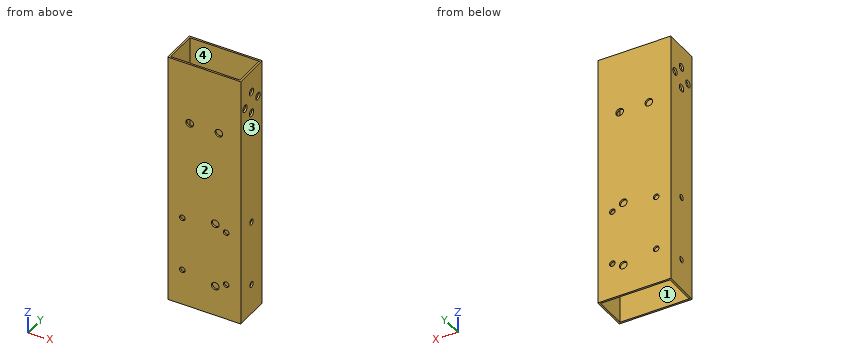
from build123d import *

# Parameters (mm, degrees)
SKETCH_1_W          = 40
SKETCH_1_H          = 20
SKETCH_1_W_2        = 38
SKETCH_1_H_2        = 18
EXTRUDE_1_DEPTH     = 140
SKETCH_2_R          = 2
SKETCH_2_R_2        = 1.55
CUT_EXTRUDE_1_DEPTH = 147.969384567
SKETCH_3_R          = 1.55
SKETCH_3_R_2        = 2.1
CUT_EXTRUDE_2_DEPTH = 147.969384567
SKETCH_4_R          = 2.1
CUT_EXTRUDE_3_DEPTH = 147.969384567


with BuildPart() as part:
    # 草图1 → 凸台-拉伸1 (new body)
    with BuildSketch(Plane.XY):
        with Locations((20, 10)):
            Rectangle(SKETCH_1_W, SKETCH_1_H)
        with Locations((20, 10)):
            Rectangle(SKETCH_1_W_2, SKETCH_1_H_2, mode=Mode.SUBTRACT)
    extrude(amount=EXTRUDE_1_DEPTH)

    # 草图2 → 切除-拉伸1 (cut, through all)
    with BuildSketch(Plane(origin=(0, 0, 0), x_dir=(0, 0, -1), z_dir=(1, 0, 0))):
        with Locations(Location((-116, 10, 0), (0, 0, 180))):
            Circle(SKETCH_2_R)
        with Locations(Location((-128, 10, 0), (0, 0, 180))):
            Circle(SKETCH_2_R)
        with Locations(Location((-16.8, 10, 0), (0, 0, 180))):
            Circle(SKETCH_2_R_2)
        with Locations(Location((-52.8, 10, 0), (0, 0, 180))):
            Circle(SKETCH_2_R_2)
        with Locations(Location((-122, 16, 0), (0, 0, 180))):
            Circle(SKETCH_2_R)
        with Locations(Location((-122, 4, 0), (0, 0, 180))):
            Circle(SKETCH_2_R)
    extrude(amount=CUT_EXTRUDE_1_DEPTH, mode=Mode.SUBTRACT)

    # 草图3 → 切除-拉伸2 (cut, through all)
    with BuildSketch(Plane(origin=(0, 0, 0), x_dir=(1, 0, 0), z_dir=(0, 1, 0))):
        with Locations(Location((8, -19.9, 0), (0, 0, 90))):
            Circle(SKETCH_3_R)
        with Locations(Location((32, -19.9, 0), (0, 0, 90))):
            Circle(SKETCH_3_R)
        with Locations(Location((32, -49.9, 0), (0, 0, 90))):
            Circle(SKETCH_3_R)
        with Locations(Location((8, -49.9, 0), (0, 0, 90))):
            Circle(SKETCH_3_R)
        with Locations(Location((26, -16.9, 0), (0, 0, 90))):
            Circle(SKETCH_3_R_2)
        with Locations(Location((26, -52.9, 0), (0, 0, 90))):
            Circle(SKETCH_3_R_2)
    extrude(amount=CUT_EXTRUDE_2_DEPTH, mode=Mode.SUBTRACT)

    # 草图4 → 切除-拉伸3 (cut, through all)
    with BuildSketch(Plane(origin=(0, 20, 0), x_dir=(1, 0, 0), z_dir=(0, 1, 0))):
        with Locations(Location((28, -106, 0), (0, 0, 270))):
            Circle(SKETCH_4_R)
        with Locations(Location((12, -106, 0), (0, 0, 270))):
            Circle(SKETCH_4_R)
    extrude(amount=-CUT_EXTRUDE_3_DEPTH, mode=Mode.SUBTRACT)


solid = part.part
The model under review builds one solid part; all positions refer to its coordinate system, in mm. Face numbers are marked on the shaded views. Give positions to 0.01 mm unless a question says otherwise; leave off trailing zeros. Write each loop counter-clockwise with the first axis right and the second up, starting at its lowest first coordinate (ties: lowest second). Pieces come first, ordered by that corner, then holes. Notation, with made-up numbers: M 55,-21.75 L 98,-21.75 A12 ccw 98,-6.75 Z; hole C -26,9 d6. An arc over 180 degrees is marked long. One line per question, with ' | ' between items. Start each with the question number.
Item 1: We need section D-D on z = 102.5. Write out the cut boundary in (x, y), plus the area to 3 significant figures.
Item 2: We need section B-B on z = 122. Write out the cut boundary in (x, y).
Item 3: For pin 1 (2 mm diameter, centred on y = 6, z = 15, fed in from -X), flat-tipped, find the tip position at first contact; note if it passes through.
Item 4: Draft analysis for pull direction X (two halves, no side actions). For the marked faces 1, 2, 3 and 4, state which applies: released by +X, released by -X, zero draft, split by the parting line, or undercut.
Item 5: We need section C-C on x = 8. Write out the cut boundary in (y, z), plus the area to 3 significant figures.
Item 6: Wall thickness on line 1 (X direction, y = 0.4, z = 106); line 2 (X direction, y = 6.5, z = 46); line 3 (X direction, y = 19.25, z = 49.9): over which ranges is each line inside the solid? List them lowest first. Write a range as from..to.
Item 7: We need section A-A on x = 36.5. Write out the cut boundary in (y, z).
Results found:
1) outline: M 0,0 L 40,0 L 40,20 L 0,20 Z; hole M 1,1 L 39,1 L 39,19 L 1,19 Z | area: 116 mm2
2) outline: M 0,0 L 40,0 L 40,2 L 39,2 L 39,1 L 1,1 L 1,2 L 0,2 Z; M 0,6 L 1,6 L 1,14 L 0,14 Z; M 0,18 L 1,18 L 1,19 L 39,19 L 39,18 L 40,18 L 40,20 L 0,20 Z; M 39,6 L 40,6 L 40,14 L 39,14 Z
3) pin 1: stops at x = 0
4) face 1: undercut | face 2: zero draft | face 3: released by +X | face 4: undercut
5) outline: M 0,0 L 1,0 L 1,18.35 L 0,18.35 Z; M 0,21.45 L 1,21.45 L 1,48.35 L 0,48.35 Z; M 0,51.45 L 1,51.45 L 1,140 L 0,140 Z; M 19,0 L 20,0 L 20,18.35 L 19,18.35 Z; M 19,21.45 L 20,21.45 L 20,48.35 L 19,48.35 Z; M 19,51.45 L 20,51.45 L 20,140 L 19,140 Z | area: 268 mm2
6) line 1: x = 0..9.9, 14.1..25.9, 30.1..40 | line 2: x = 0..1, 39..40 | line 3: x = 0..6.45, 9.55..30.45, 33.55..40
7) outline: M 0,0 L 1,0 L 1,140 L 0,140 Z; M 19,0 L 20,0 L 20,140 L 19,140 Z
